The model under review builds one solid part; all positions refer to its coordinate system, in mm. A direction names the side the tool comes from. Coordinates: 2 decimals unless noted, no trailing zeros. Write each loop counter-clockwise with the first axis right and the second up, starting at its lowest first coordinate (ties: lowest second). Pieces come first, ordered by that corner, then holes. Notation, with made-up numbers: (16, -39) - (62, -39) arc R20 ccw to (62, -8) - close; hole circle Ø9 at (-22, -15.75). An arc over 180 degrees is marked (long way). Put each result on its own line as item: value. Start each with the question number.
Item 1: Consider section B-B on y = -41.5. Give the boundary of the cut face in (x, z).
Item 2: To check wall thickness, follow L1, parallel to Z at x = -99, y = -35; L2, parallel to X at y = -1, z = 11.25; L3, parallel to Y at x = -130, z = 7.25. State the ranges of each line that lie inside material, in increasing order. Write a range as [from, to].
Item 3: For pin 1 (22.5 mm diameter, centred on x = -89, y = -56, fed in from +Z); pin 2 (8 mm diameter, centred on x = -16, z = 17.5, fed in from +Y); pin 3 (1.5 mm diameter, centred on y = -59, z = 8.5, fed in from -X), all flat-tipped, find the tip position at first contact; note any pin that passes through.
Item 4: Mouldability with a two-part tool opening along X and no side actions: class faces 1 (the face through (-160.6, -51.1, 2.5)), 2 (the face through (-2.17, -9.76, 7.4)), 3 (the face through (28, -76, 5)) as pulls with the +X half, pulls with the -X half, needs draft (parallel to the pull), parting line crosses it, or undercut.
Item 5: Consider section A-A on x = -106. Give the boundary of the cut face in (y, z), then the cut area to 3 significant figures.
Item 6: Machinability: for faces 4 (the face through (-71, -59, 7)), 5 (the face through (7.3, -7.3, 15)), 6 (the face through (-91, -70, 5)), 7 (the face through (28, 11.58, 9.86)), 8 (the face through (-166, -76, 7)), which of the approach directions +Z, -Z, +X, -X, +Y, -Y give a long, thin tool a straight path to every point of the face, cutting with its end or side? Answer none if there is none.
```python
from build123d import *

# Parameters (mm, degrees)
SKETCH_1_R      = 4
EXTRUDE_1_DEPTH = 10
EXTRUDE_2_DEPTH = 5
SKETCH_1_4_R    = 17
SKETCH_1_4_R_2  = 10
EXTRUDE_3_DEPTH = 15
SKETCH_1_5_R    = 38
SKETCH_1_5_R_2  = 5
SKETCH_1_5_R_3  = 17
EXTRUDE_4_DEPTH = 20


with BuildPart() as part:
    # Sketch 1 → Extrude 1 (new body)
    with BuildSketch(Plane.XY):
        with BuildLine():
            Line((-198, -90), (-121, -90))
            Line((-121, -90), (-121, -50))
            ThreePointArc((-121, -50), (-106, -35), (-91, -50))
            Line((-91, -50), (-91, -90))
            Line((-91, -90), (52, -90))
            ThreePointArc((52, -90), (47.899494937, -80.100505063), (38, -76))
            Line((38, -76), (17.320508076, -76))
            ThreePointArc((17.320508076, -76), (8.660254038, -71), (8.660254038, -61))
            Line((8.660254038, -61), (32.908965344, -19))
            ThreePointArc((32.908965344, -19), (15.44850963, -34.718057984), (-7.916666667, -37.166199549))
            ThreePointArc((-7.916666667, -37.166199549), (-0.863668952, -42.881381106), (-1.339745962, -51.946778377))
            Line((-1.339745962, -51.946778377), (-11.762778326, -70))
            ThreePointArc((-11.762778326, -70), (-16.155083171, -74.392304845), (-22.155083171, -76))
            Line((-22.155083171, -76), (-63, -76))
            ThreePointArc((-63, -76), (-68.656854249, -73.656854249), (-71, -68))
            Line((-71, -68), (-71, -50))
            ThreePointArc((-71, -50), (-106, -15), (-141, -50))
            Line((-141, -50), (-141, -68))
            ThreePointArc((-141, -68), (-143.343145751, -73.656854249), (-149, -76))
            Line((-149, -76), (-184, -76))
            ThreePointArc((-184, -76), (-193.899494937, -80.100505063), (-198, -90))
        make_face()
        with Locations((-130, -50)):
            Circle(SKETCH_1_R, mode=Mode.SUBTRACT)
        with Locations((-82, -50)):
            Circle(SKETCH_1_R, mode=Mode.SUBTRACT)
        with Locations((-122.970562748, -33.029437252)):
            Circle(SKETCH_1_R, mode=Mode.SUBTRACT)
        with Locations((-89.029437252, -33.029437252)):
            Circle(SKETCH_1_R, mode=Mode.SUBTRACT)
        with Locations((-106, -26)):
            Circle(SKETCH_1_R, mode=Mode.SUBTRACT)
    extrude(amount=EXTRUDE_1_DEPTH)

    # Sketch 1_3 → Extrude 2 (add)
    with BuildSketch(Plane.XY):
        with BuildLine():
            Line((-128.966962921, -23.589422305), (-193.186785168, -79.435768922))
            ThreePointArc((-193.186785168, -79.435768922), (-188.904118927, -76.887043905), (-184, -76))
            Line((-184, -76), (-149, -76))
            ThreePointArc((-149, -76), (-143.343145751, -73.656854249), (-141, -68))
            Line((-141, -68), (-141, -50))
            ThreePointArc((-141, -50), (-137.849989813, -35.488688933), (-128.966962921, -23.589422305))
        make_face()
        with BuildLine():
            ThreePointArc((-36.043919772, 12.034776584), (-59.305035094, -14.640262917), (-94.625446436, -16.899856024))
            ThreePointArc((-94.625446436, -16.899856024), (-77.512201079, -29.666645318), (-71, -50))
            Line((-71, -50), (-71, -68))
            ThreePointArc((-71, -68), (-68.656854249, -73.656854249), (-63, -76))
            Line((-63, -76), (-22.155083171, -76))
            ThreePointArc((-22.155083171, -76), (-16.155083171, -74.392304845), (-11.762778326, -70))
            Line((-11.762778326, -70), (-1.339745962, -51.946778377))
            ThreePointArc((-1.339745962, -51.946778377), (-0.863668952, -42.881381106), (-7.916666667, -37.166199549))
            ThreePointArc((-7.916666667, -37.166199549), (-32.989654486, -18.859551874), (-36.043919772, 12.034776584))
        make_face()
    extrude(amount=EXTRUDE_2_DEPTH)



with BuildPart() as body_2:
    # Sketch 1_4 → Extrude 3 (new body)
    with BuildSketch(Plane.XY):
        Circle(SKETCH_1_4_R)
        Circle(SKETCH_1_4_R_2, mode=Mode.SUBTRACT)
    extrude(amount=EXTRUDE_3_DEPTH)


with BuildPart() as part_1:
    add(part.part)

    add(body_2.part)  # Extrude 4 merges body 2
    # Sketch 1_5 → Extrude 4 (add)
    with BuildSketch(Plane.XY):
        with Locations(Location((0, 0, 0), (0, 0, 161.536247512))):
            Circle(SKETCH_1_5_R)
        with Locations((-13.5, 23.382685902)):
            Circle(SKETCH_1_5_R_2, mode=Mode.SUBTRACT)
        with Locations((-23.382685902, 13.5)):
            Circle(SKETCH_1_5_R_2, mode=Mode.SUBTRACT)
        with Locations((-27, 0)):
            Circle(SKETCH_1_5_R_2, mode=Mode.SUBTRACT)
        with Locations((-23.382685902, -13.5)):
            Circle(SKETCH_1_5_R_2, mode=Mode.SUBTRACT)
        with Locations((-13.5, -23.382685902)):
            Circle(SKETCH_1_5_R_2, mode=Mode.SUBTRACT)
        with Locations((0, -27)):
            Circle(SKETCH_1_5_R_2, mode=Mode.SUBTRACT)
        with Locations((13.5, -23.382685902)):
            Circle(SKETCH_1_5_R_2, mode=Mode.SUBTRACT)
        with Locations((23.382685902, -13.5)):
            Circle(SKETCH_1_5_R_2, mode=Mode.SUBTRACT)
        with Locations((27, 0)):
            Circle(SKETCH_1_5_R_2, mode=Mode.SUBTRACT)
        with Locations((23.382685902, 13.5)):
            Circle(SKETCH_1_5_R_2, mode=Mode.SUBTRACT)
        with Locations((13.5, 23.382685902)):
            Circle(SKETCH_1_5_R_2, mode=Mode.SUBTRACT)
        with Locations((0, 27)):
            Circle(SKETCH_1_5_R_2, mode=Mode.SUBTRACT)
        Circle(SKETCH_1_5_R_3, mode=Mode.SUBTRACT)
    extrude(amount=EXTRUDE_4_DEPTH)


solid = part_1.part
```
Report:
1. outline: (-149.56, 0) - (-118.36, 0) - (-118.36, 10) - (-139.95, 10) - (-139.95, 5) - (-149.56, 5) - close; (-93.64, 0) - (19.92, 0) - (19.92, 10) - (-1.61, 10) - (-1.61, 5) - (-72.05, 5) - (-72.05, 10) - (-93.64, 10) - close
2. L1: [0, 10]
2. L2: [-37.99, -31.9], [-22.1, -9.95], [9.95, 22.1], [31.9, 37.99]
2. L3: [-90, -54], [-46, -24.52]
3. pin 1: z = 10
3. pin 2: y = 36.06
3. pin 3: x = -141
4. face 1: pulls with the -X half
4. face 2: undercut
4. face 3: needs draft
5. outline: (-35, 0) - (-30, 0) - (-30, 10) - (-35, 10) - close; (-22, 0) - (-15, 0) - (-15, 10) - (-22, 10) - close
5. area: 120 mm²
6. face 4: +Z, +Y
6. face 5: +Z
6. face 6: +Z, -Z, -Y
6. face 7: +Z, -Z
6. face 8: +Z, -X, +Y
